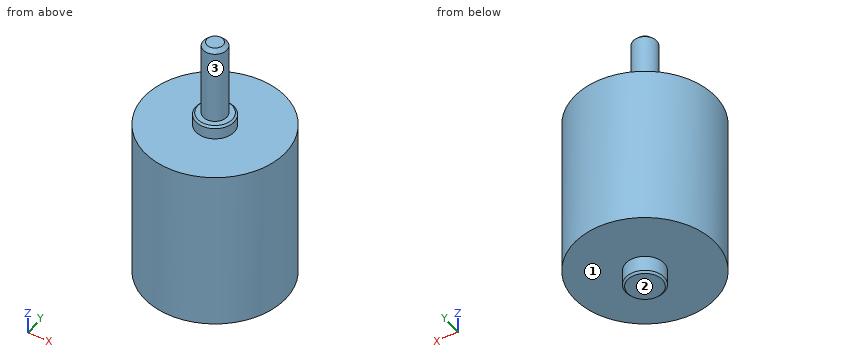
```python
from build123d import *

# Parameters (mm, degrees)
CHAMFER1_SIZE = 1.016
CHAMFER2_SIZE = 0.508


with BuildPart() as part:
    # Sketch1 → Revolve1 (revolve)
    with BuildSketch(Plane(origin=(0, 0, 0), x_dir=(0, 0, -1), z_dir=(1, 0, 0)), mode=Mode.PRIVATE) as revolve1_sk:
        Polygon((0, 0), (0, 3.175), (21, 3.175), (21, 5.1689), (24.556, 5.1689), (24.556, 19.05), (68.134749365, 19.05), (68.134749365, 5.1689), (72.7964, 5.1689), (72.7964, 0), align=None)
    revolve(revolve1_sk.sketch.rotate(Axis((0, 0, 0), (0, 0, -1)), 90), axis=Axis((0, 0, 0), (0, 0, -1)))

    # Chamfer1
    chamfer1_edges = [part.edges().sort_by_distance(p)[0] for p in [
        (-3.175, 0, 0),
    ]]
    chamfer(chamfer1_edges, length=CHAMFER1_SIZE)

    # Chamfer2
    chamfer2_edges = [part.edges().sort_by_distance(p)[0] for p in [
        (-5.1689, 0, -72.7964),
        (-5.1689, 0, -21),
    ]]
    chamfer(chamfer2_edges, length=CHAMFER2_SIZE)


solid = part.part
```
Design review of the part built by this model. Coordinates are the model's own, in mm. Face numbers are marked on the shaded views. A direction names the side the tool comes from. Coordinates: 2 decimals unless noted, no trailing zeros. Order: outer loops, then holes, each group sorted by start corner. A loop starts at its lowest first (then second) coordinate and runs counter-clockwise, first axis right, second up. Notation, with made-up numbers: M 26.25,13 L 48.25,13 A18 ccw 48.25,42 Z; hole C 9,47.5 d4. An arc over 180 degrees is marked long. Answer as a JSON object with one key per item and string values. Group by question number.
1) Add section C-C, the plane z = -31.5. Write out the cut boundary in (x, y), then the cut area to 3 significant figures.
2) For pin 1 (4 mm diameter, centred on x = 9.5, z = -61.5, fed in from -Y); pin 2 (4.5 mm diameter, centred on x = -0.5, y = -1, fed in from +Z); pin 3 (1.5 mm diameter, centred on x = 3.5, z = -45, fed in from -Y); pin 4 (5 mm diameter, centred on x = 11, y = 5.5, fed in from +Z), all flat-tipped, find the tip position at first contact; note any pin that passes through.
3) Add section A-A, the plane y = 0. Write out the cut boundary in (x, z) (3 decimals).
4) Wall thickness on L1, parallel to Z at x = 17, y = 1.5; L2, parallel to Y at x = 16, z = -53.5: over which ranges is each line inside the solid? List them lowest first.
5) Add section D-D, the plane y = -11. Write out the cut boundary in (x, z).
6) Tool access review of the marked faces 1, 2 and 3: name each direction out of +Z, -Z, +X, -X, +Y, -Y from which nothing blocks a thin tool from reaching the whole face with its end or side.
Computed values:
{
 "1": {"outline": "C 0,0 d38.1", "area": "1,140 mm^2"},
 "2": {"pin 1": "stops at y = -17.51", "pin 2": "stops at z = 0", "pin 3": "stops at y = -18.85", "pin 4": "stops at z = -24.56"},
 "3": {"outline": "M -19.05,-68.135 L -5.169,-68.135 L -5.169,-72.288 L -4.661,-72.796 L 4.661,-72.796 L 5.169,-72.288 L 5.169,-68.135 L 19.05,-68.135 L 19.05,-24.556 L 5.169,-24.556 L 5.169,-21.508 L 4.661,-21 L 3.175,-21 L 3.175,-1.016 L 2.159,0 L -2.159,0 L -3.175,-1.016 L -3.175,-21 L -4.661,-21 L -5.169,-21.508 L -5.169,-24.556 L -19.05,-24.556 Z"},
 "4": {"L1": "z = -68.13 to -24.56", "L2": "y = -10.34 to 10.34"},
 "5": {"outline": "M -15.55,-68.13 L 15.55,-68.13 L 15.55,-24.56 L -15.55,-24.56 Z"},
 "6": {"face 1": "-Z", "face 2": "-Z, +X, -X, +Y, -Y", "face 3": "+Z"}
}
